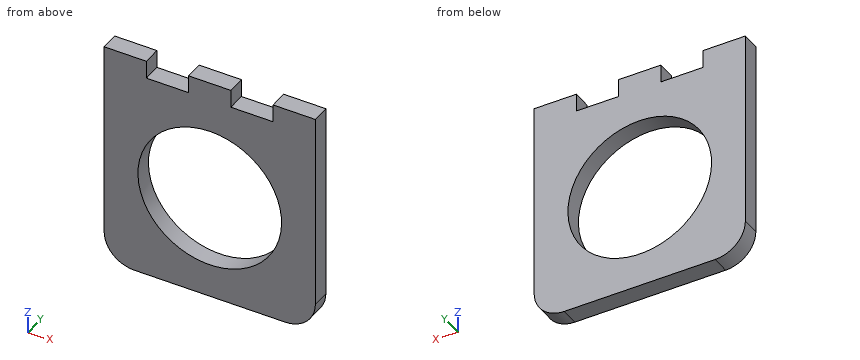
```python
from build123d import *

# Parameters (mm, degrees)
SKETCH2_W           = 35
SKETCH2_H           = 38
BOSS_EXTRUDE1_DEPTH = 3
SKETCH3_R           = 11.9
CUT_EXTRUDE1_DEPTH  = 3
FILLET1_R           = 5
FILLET2_R           = 5
SKETCH4_W           = 7
SKETCH4_H           = 3
CUT_EXTRUDE2_DEPTH  = 3
LPATTERN1_COUNT     = 2
LPATTERN1_PITCH     = 14


with BuildPart() as part:
    # Sketch2 → Boss-Extrude1 (new body)
    with BuildSketch(Plane(origin=(0, 0, 0), x_dir=(1, 0, 0), z_dir=(0, 1, 0))):
        Rectangle(SKETCH2_W, SKETCH2_H)
    extrude(amount=BOSS_EXTRUDE1_DEPTH)

    # Sketch3 → Cut-Extrude1 (cut)
    with BuildSketch(Plane(origin=(0, 3, 0), x_dir=(1, 0, 0), z_dir=(0, 1, 0))):
        with Locations(Location((0, 1.5, 0), (0, 0, 270))):
            Circle(SKETCH3_R)
    extrude(amount=-CUT_EXTRUDE1_DEPTH, mode=Mode.SUBTRACT)

    # Fillet1
    fillet1_edges = [part.edges().sort_by_distance(p)[0] for p in [
        (17.5, 1.5, -19),
    ]]
    fillet(fillet1_edges, radius=FILLET1_R)

    # Fillet2
    fillet2_edges = [part.edges().sort_by_distance(p)[0] for p in [
        (-17.5, 1.5, -19),
    ]]
    fillet(fillet2_edges, radius=FILLET2_R)

    # Sketch4 → Cut-Extrude2 (cut)
    with BuildSketch(Plane(origin=(0, 3, 0), x_dir=(1, 0, 0), z_dir=(0, 1, 0))):
        with Locations((-7, -17.5)):
            Rectangle(SKETCH4_W, SKETCH4_H)
    cut_extrude2 = extrude(amount=-CUT_EXTRUDE2_DEPTH, mode=Mode.SUBTRACT)

    # LPattern1: Cut-Extrude2 ×2
    with Locations(*[(i * LPATTERN1_PITCH, 0, 0) for i in range(1, LPATTERN1_COUNT)]):
        add(cut_extrude2, mode=Mode.SUBTRACT)


solid = part.part
```
Work out the finished part from the listing and answer in its coordinate system (mm). Give positions to 0.01 mm unless a question says otherwise; leave off trailing zeros. Order: outer loops, then holes, each group sorted by start corner. A loop starts at its lowest first (then second) coordinate and runs counter-clockwise, first axis right, second up. Notation, with made-up numbers: (76, -31.75) -> (89, -31.75) arc R22 ccw to (89, 3.25) -> close; hole circle Ø5 at (-34, -32.75). An arc over 180 degrees is marked (long way). Answer as CSV lines item,"result". Start each with the question number.
(1) Section B-B, the plane x = 0 is taken. Write down the section's boundary in (y, z).
(2) Section D-D, the plane x = 15.5 is taken. Write down the section's boundary in (y, z).
(3) Section C-C, the plane y = 2.2 is taken. Write down the section's boundary in (x, z), plus the area to 3 significant figures.
(4) This flat-tipped pin is pushed along its axis until it touches: pin 1 Ø1 at (x, y) = (-9.5, 2) entering from +Z. Where does it stop, or does it pass through?
(5) Section A-A, the plane z = -1.5 is taken. Write down the section's boundary in (x, y).
(6) Consider line 1 along X through (y, z) = (0.4, 17); line 2 along X through (y, z) = (2.75, -2); line 3 along Z through (x, y) = (1, 1). Determine where each line is inside the solid, lowest interval first.
Entries:
1,outline,"(0, -19) -> (3, -19) -> (3, -13.4) -> (0, -13.4) -> close; (0, 10.4) -> (3, 10.4) -> (3, 19) -> (0, 19) -> close"
2,outline,"(0, -18) -> (3, -18) -> (3, 19) -> (0, 19) -> close"
3,outline,"(-17.5, -14) arc R5 ccw to (-12.5, -19) -> (12.5, -19) arc R5 ccw to (17.5, -14) -> (17.5, 19) -> (10.5, 19) -> (10.5, 16) -> (3.5, 16) -> (3.5, 19) -> (-3.5, 19) -> (-3.5, 16) -> (-10.5, 16) -> (-10.5, 19) -> (-17.5, 19) -> close; hole circle Ø23.8 at (0, -1.5)"
3,area,"832 mm²"
4,pin 1,"z = 16"
5,outline,"(-17.5, 0) -> (-11.9, 0) -> (-11.9, 3) -> (-17.5, 3) -> close; (11.9, 0) -> (17.5, 0) -> (17.5, 3) -> (11.9, 3) -> close"
6,line 1,"-17.5 to -10.5, -3.5 to 3.5, 10.5 to 17.5"
6,line 2,"-17.5 to -11.89, 11.89 to 17.5"
6,line 3,"-19 to -13.36, 10.36 to 19"
